Autodesk Inventor part; units mm, degrees
ref_plane "YZ Plane" through (0, 0, 0) normal (1, 0, 0) x (0, 1, 0)
ref_plane "XZ Plane" through (0, 0, 0) normal (0, 1, 0) x (-1, 0, 0)
ref_plane "XY Plane" through (0, 0, 0) normal (0, 0, 1) x (1, 0, 0)
sketch "Szkic1" plane through (0, 0, 0) normal (0, 0, 1) x (1, 0, 0)
  point P0 (0, 0)
sketch "Szkic2" plane through (0, 0, 0) normal (0, 1, 0) x (-1, 0, 0)
  line L0 (30, 5) -> (-30, 5)
  line L1 (-30, 5) -> (-30, -5)
  line L2 (-30, -5) -> (30, -5)
  line L3 (30, -5) -> (30, 5)
  line L4 (13.3205, 0) -> (-15.9073, 0) construction
  line L5 (0, 22.8583) -> (0, -40.0607) construction
  point P0 (0, 0)
  dimension "d0" = 10
  dimension "d1" = 60
extrude "Wyciągnięcie proste1" add sketch "Szkic2" along normal blind 5
sketch "Szkic3" plane through (0, 5, 0) normal (0, 1, 0) x (1, 0, 0)
  line L0 (-30, 5) -> (-30, -5)
  line L1 (30, 5) -> (-30, 5)
  line L2 (-30, -5) -> (-10, -5)
  line L3 (-10, -5) -> (-10, 5)
  line L4 (-10, 5) -> (-30, 5)
  line L5 (-30, 5) -> (-30, -5)
  line L6 (30, -5) -> (10, -5)
  line L7 (10, -5) -> (10, 5)
  line L8 (10, 5) -> (30, 5)
  line L9 (30, 5) -> (30, -5)
  line L10 (0, 41.547) -> (0, -40.407) construction
  circle A0 centre (0, 0) radius 1.5
  dimension "d4" = 20
  dimension "d5" = 20
  dimension "d6" = 3
extrude "Wyciągnięcie proste2" add sketch "Szkic3" along normal blind 5
sketch "Szkic4" plane through (0, 10, 0) normal (0, 1, 0) x (1, 0, 0)
  line L0 (0, 14.0263) -> (0, -15.9036) construction
  line L1 (-30, 5) -> (-30, -5)
  point P0 (0, 0)
  point P1 (-20, 0)
  point P2 (20, 0)
  dimension "d9" = 10
hole "Otwór1" at (-20, 10, 0) at (20, 10, 0) direction (0, -1, 0) diameter 4.134 depth 5 tip angle 118
properties part number "środek"
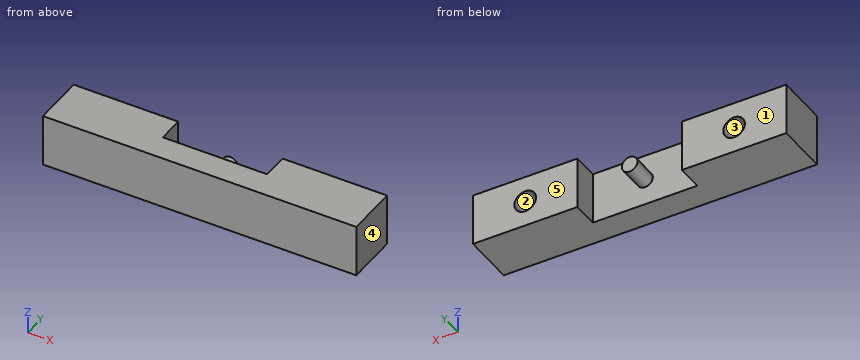
Verification items for the finished model (mm, model axes). Face numbers are marked on the shaded views. A direction names the side the tool comes from. Coordinates: 2 decimals unless noted, no trailing zeros. Order: outer loops, then holes, each group sorted by start corner. A loop starts at its lowest first (then second) coordinate and runs counter-clockwise, first axis right, second up. Notation, with made-up numbers: (85, 70) -> (128, 70) arc R11 cw to (128, 77) -> close; hole circle Ø1 at (54.5, -9). An arc over 180 degrees is marked (long way). Answer as CSV lines item,"result". Start each with the question number.
1) Material ranges on L1, parallel to X at y = 8, z = 0; L2, parallel to X at y = 8.25, z = -2.5; L3, parallel to Z at x = -20, y = 6.35, recorded low to high. Write a range as [from, to].
2) Cross-section at C-C, the plane y = 4.5. Record the boundary of the cut face in (x, z), then the cut area to 3 significant figures.
3) Set-up check for the marked faces 1 and 2: record each of +Z, -Z, +X, -X, +Y, -Y from which the full face is reachable in a straight line by a thin tool's end or side.
4) Gauge pin test, flat ends, axial feed: pin 1 Ø3.5 at (x, z) = (-20, 0) entering from +Y; pin 2 Ø3 at (x, z) = (8.5, -1) entering from -Y. Record the tip position at first contact, or that the pin passes through.
5) Cross-section at B-B, the plane x = 0. Record the boundary of the cut face in (y, z).
6) Cross-section at A-A, the plane z = 3.5. Record the boundary of the cut face in (x, y), then the cut area to 3 significant figures.
7) Release check for a two-part mould opening along X. For the marked faces 3, 4 and 5 record: released by +X, released by -X, zero draft, split by the parting line, or undercut.
Conclusion:
1,L1,"x = [-30, -22.07], [-17.93, -10], [-1.5, 1.5], [10, 17.93], [22.07, 30]"
1,L2,"x = [-30, -10], [10, 30]"
1,L3,"z = [-5, -2.07], [2.07, 5]"
2,outline,"(-30, -5) -> (30, -5) -> (30, 5) -> (-30, 5) -> close; hole circle Ø2.47 at (-20, 0); hole circle Ø2.47 at (20, 0)"
2,area,"590 mm²"
3,face 1,"+Z, -Z, +X, -X, +Y"
3,face 2,"+Y"
4,pin 1,"stops at y = 4.81"
4,pin 2,"stops at y = 0"
5,outline,"(0, -5) -> (5, -5) -> (5, -1.5) -> (10, -1.5) -> (10, 1.5) -> (5, 1.5) -> (5, 5) -> (0, 5) -> close"
6,outline,"(-30, 0) -> (30, 0) -> (30, 10) -> (10, 10) -> (10, 5) -> (-10, 5) -> (-10, 10) -> (-30, 10) -> close"
6,area,"500 mm²"
7,face 3,"undercut"
7,face 4,"released by +X"
7,face 5,"zero draft"
